```python
from build123d import *

# Parameters (mm, degrees)
F0_R     = 1.6169626647
F1_DEPTH = 3.048


with BuildPart() as f1:
    # F0 (on Front) → F1 (new body)
    with BuildSketch(Plane.XZ):
        with BuildLine():
            ThreePointArc((-63.3394401935, 51.5408627689), (-60.5300601386, 44.7584193386), (-53.7476167083, 41.9490392837))
            ThreePointArc((-53.7476167083, 41.9490392837), (-46.9651732779, 44.7584193386), (-44.1557932231, 51.5408627689))
            ThreePointArc((-44.1557932231, 51.5408627689), (-53.7476167083, 61.1326862541), (-63.3394401935, 51.5408627689))
        make_face()
        with BuildLine():
            ThreePointArc((-50.3500356436, 51.5408627689), (-51.3451640978, 49.1384101584), (-53.7476167083, 48.1432817042))
            ThreePointArc((-53.7476167083, 48.1432817042), (-56.1500693187, 53.9433153794), (-50.3500356436, 51.5408627689))
        make_face(mode=Mode.SUBTRACT)
        with BuildLine():
            ThreePointArc((-44.1557932231, 51.5408627689), (-46.9651732779, 44.7584193386), (-53.7476167083, 41.9490392837))
            Line((-53.7476167083, 41.9490392837), (-53.7476167083, 17.560091))
            ThreePointArc((-53.7476167083, 17.560091), (-43.320354495, 13.6211561996), (-38.1016313362, 3.7718956578))
            Line((-38.1016313362, 3.7718956578), (-44.1557932231, 51.5408627689))
        make_face()
        with BuildLine():
            Line((-53.7476167083, 17.560091), (-53.7476167083, 41.9490392837))
            ThreePointArc((-53.7476167083, 41.9490392837), (-60.5300601386, 44.7584193386), (-63.3394401935, 51.5408627689))
            Line((-63.3394401935, 51.5408627689), (-69.3936021245, 3.7718953097))
            ThreePointArc((-69.3936021245, 3.7718953097), (-64.1748790532, 13.6211560835), (-53.7476167083, 17.560091))
        make_face()
        with Locations((-55.8080822229, 37.366181612)):
            Circle(F0_R, mode=Mode.SUBTRACT)
        with BuildLine():
            ThreePointArc((-38.1016313362, 3.7718956578), (-43.320354495, 13.6211561996), (-53.7476167083, 17.560091))
            Line((-53.7476167083, 17.560091), (-53.7476167083, 3.3594787524))
            ThreePointArc((-53.7476167083, 3.3594787524), (-52.6370840671, 2.8994810709), (-52.1770863857, 1.7889484297))
            ThreePointArc((-52.1770863857, 1.7889484297), (-52.6370840671, 0.6784157886), (-53.7476167083, 0.2184181071))
            Line((-53.7476167083, 0.2184181071), (-53.7476167083, -13.9821941405))
            ThreePointArc((-53.7476167083, -13.9821941405), (-42.5957348498, -9.3629334288), (-37.976474138, 1.7889484297))
            ThreePointArc((-37.976474138, 1.7889484297), (-38.0077945376, 2.78239496), (-38.1016313362, 3.7718956578))
        make_face()
        with BuildLine():
            Line((-53.7476167083, 3.3594787524), (-53.7476167083, 17.560091))
            ThreePointArc((-53.7476167083, 17.560091), (-64.1748790532, 13.6211560835), (-69.3936021245, 3.7718953097))
            ThreePointArc((-69.3936021245, 3.7718953097), (-65.5798243621, -8.6383139152), (-53.7476167083, -13.9821941405))
            Line((-53.7476167083, -13.9821941405), (-53.7476167083, 0.2184181071))
            ThreePointArc((-53.7476167083, 0.2184181071), (-55.3181470309, 1.7889484297), (-53.7476167083, 3.3594787524))
        make_face()
        with BuildLine():
            Line((-37.6235873609, 0), (-38.1016313362, 3.7718956578))
            ThreePointArc((-38.1016313362, 3.7718956578), (-38.0077945376, 2.78239496), (-37.976474138, 1.7889484297))
            ThreePointArc((-37.976474138, 1.7889484297), (-42.5957348498, -9.3629334288), (-53.7476167083, -13.9821941405))
            Line((-53.7476167083, -13.9821941405), (-53.7476167083, -54.9663756517))
            ThreePointArc((-53.7476167083, -54.9663756517), (-48.1772102832, -57.2737135409), (-45.869872394, -62.844119966))
            Line((-45.869872394, -62.844119966), (-16.1001367542, -62.844119966))
            ThreePointArc((-16.1001367542, -62.844119966), (-13.8006404187, -57.278812686), (-8.2434529492, -54.9597620295))
            Line((-8.2434529492, -54.9597620295), (-35.7097443, -55.0563386246))
            ThreePointArc((-35.7097443, -55.0563386246), (-41.7018969318, -52.3629945232), (-43.6213969554, -46.0800401807))
            Line((-43.6213969554, -46.0800401807), (-37.6235873609, 0))
        make_face()
        with BuildLine():
            ThreePointArc((-53.7476167083, -13.9821941405), (-65.5798243621, -8.6383139152), (-69.3936021245, 3.7718953097))
            Line((-69.3936021245, 3.7718953097), (-69.8716460556, 0))
            Line((-69.8716460556, 0), (-61.5594655419, -63.8609155613))
            ThreePointArc((-61.5594655419, -63.8609155613), (-59.6666078048, -57.6456201939), (-53.7476167083, -54.9663756517))
            Line((-53.7476167083, -54.9663756517), (-53.7476167083, -13.9821941405))
        make_face()
        with BuildLine():
            Line((-53.7476167083, -59.5422655519), (-53.7476167083, -54.9663756517))
            ThreePointArc((-53.7476167083, -54.9663756517), (-59.6666078048, -57.6456201939), (-61.5594655419, -63.8609155613))
            ThreePointArc((-61.5594655419, -63.8609155613), (-58.991522279, -68.7229217017), (-53.868886638, -70.7209308109))
            Line((-53.868886638, -70.7209308109), (-53.6263467786, -70.7209308109))
            ThreePointArc((-53.6263467786, -70.7209308109), (-48.1344986363, -68.371484708), (-45.869872394, -62.844119966))
            Line((-45.869872394, -62.844119966), (-50.4457622942, -62.844119966))
            ThreePointArc((-50.4457622942, -62.844119966), (-56.082380355, -65.1788836127), (-53.7476167083, -59.5422655519))
        make_face()
        with BuildLine():
            Line((-16.1001367542, -62.844119966), (-45.869872394, -62.844119966))
            ThreePointArc((-45.869872394, -62.844119966), (-48.1344986363, -68.371484708), (-53.6263467786, -70.7209308109))
            Line((-53.6263467786, -70.7209308109), (-8.5617351981, -70.7209308109))
            ThreePointArc((-8.5617351981, -70.7209308109), (-13.9118653342, -68.2955337071), (-16.1001367542, -62.844119966))
        make_face()
        with BuildLine():
            Line((-53.6263467786, -70.7209308109), (-53.868886638, -70.7209308109))
            ThreePointArc((-53.868886638, -70.7209308109), (-53.7476167083, -70.7218642803), (-53.6263467786, -70.7209308109))
        make_face()
        with BuildLine():
            ThreePointArc((-0.3313234028, -62.844119966), (-2.6504227985, -57.2592096259), (-8.2434529492, -54.9597620295))
            ThreePointArc((-8.2434529492, -54.9597620295), (-13.8006404187, -57.278812686), (-16.1001367542, -62.844119966))
            ThreePointArc((-16.1001367542, -62.844119966), (-13.9118653342, -68.2955337071), (-8.5617351981, -70.7209308109))
            Line((-8.5617351981, -70.7209308109), (-7.8697249589, -70.7209308109))
            ThreePointArc((-7.8697249589, -70.7209308109), (-2.5195948228, -68.2955337071), (-0.3313234028, -62.844119966))
        make_face()
        with BuildLine():
            ThreePointArc((-5.0356472554, -62.844119966), (-8.2157300785, -66.0242027891), (-11.3958129016, -62.844119966))
            ThreePointArc((-11.3958129016, -62.844119966), (-8.2157300785, -59.6640371429), (-5.0356472554, -62.844119966))
        make_face(mode=Mode.SUBTRACT)
        with BuildLine():
            Line((-7.8697249589, -70.7209308109), (-8.5617351981, -70.7209308109))
            ThreePointArc((-8.5617351981, -70.7209308109), (-8.2157300785, -70.7285266418), (-7.8697249589, -70.7209308109))
        make_face()
        with BuildLine():
            ThreePointArc((-45.869872394, -62.844119966), (-48.1772102832, -57.2737135409), (-53.7476167083, -54.9663756517))
            Line((-53.7476167083, -54.9663756517), (-53.7476167083, -59.5422655519))
            ThreePointArc((-53.7476167083, -59.5422655519), (-51.4128530616, -60.5093563193), (-50.4457622942, -62.844119966))
            Line((-50.4457622942, -62.844119966), (-45.869872394, -62.844119966))
        make_face()
    extrude(amount=F1_DEPTH)


solid = f1.part
```
Verification items for the finished model (mm, model axes). Round coordinates to 2 decimals unless told otherwise and drop trailing zeros. Loops run counter-clockwise (first coordinate to the right, second up) from the corner with the lowest first, then second, coordinate; pieces in that order, holes last. Notation, with made-up numbers: (-31, 59.25) -> (0, 59.25) arc R21 cw to (0, 76.25) -> close; hole circle Ø8 at (82, 16). An arc over 180 degrees is marked (long way). Answer as a JSON object with one key per item and string values.
Q1. Draft check along X on faces 1 (the flat face through (-40.664, -1.503, -23.363)), 2 (the flat face through (-51, 0, -4)), 3 (the cylindrical face through (-54.314, -1.503, 36.747)). Enter one of: pulls with the +X half, pulls with the -X half, needs draft (parallel to the pull), parting line crosses it, or undercut.
Data:
{"face 1": "pulls with the +X half", "face 2": "needs draft", "face 3": "undercut"}
Q2. Section check B-B (x = -15.5). Record the boundary of the cut face in (y, z), then the cut area to 3 significant figures.
Data:
{"outline": "(-3.05, -70.72) -> (0, -70.72) -> (0, -54.99) -> (-3.05, -54.99) -> close", "area": "48.0 mm2"}
Q3. Scan lines: line 1 (Z direction, x = -32.5, y = -2.45); line 2 (X direction, y = -0.4, z = 1); line 3 (Z direction, x = -55.5, y = -1.8). Record each from-to range of solid material in increasing order. Write a range as from..to.
Data:
{"line 1": "z = -70.72..-55.05", "line 2": "x = -69.74..-55.11, -52.39..-37.75", "line 3": "z = -70.52..-65.64, -60.05..35.78, 38.95..48.63, 54.45..60.97"}
Q4. Section check A-A (y = -0.7). Record the boundary of the cut face in (x, z), then the cut area to 3 significant figures.
Data:
{"outline": "(-69.87, 0) -> (-61.56, -63.86) arc R7.88 ccw to (-53.63, -70.72) -> (-8.56, -70.72) arc R7.88 ccw (long way) to (-8.24, -54.96) -> (-35.71, -55.06) arc R7.95 cw to (-43.62, -46.08) -> (-37.62, 0) -> (-44.16, 51.54) arc R9.59 ccw to (-63.34, 51.54) -> close; hole circle Ø3.23 at (-55.81, 37.37); hole circle Ø6.8 at (-53.75, 51.54); hole circle Ø6.6 at (-53.75, -62.84); hole circle Ø3.14 at (-53.75, 1.79); hole circle Ø6.36 at (-8.22, -62.84)", "area": "3,680 mm2"}
Q5. Go/stop test with flat-tipped pins: P1, Ø1.5, axis at x = -40, y = -1.5, coming from the -Z side; P2, Ø8, axis at x = -37.5, z = -14, coming from the +Y side. Record where each tip stops, or that it passes through.
Data:
{"P1": "stops at z = -70.72", "P2": "stops at y = 0"}
Q6. Section check C-C (z = 21). Record the boundary of the cut face in (x, y), then the cut area to 3 significant figures.
Data:
{"outline": "(-67.21, -3.05) -> (-40.29, -3.05) -> (-40.29, 0) -> (-67.21, 0) -> close", "area": "82.1 mm2"}
